```python
from build123d import *

# Parameters (mm, degrees)
PAD_DEPTH    = 22
SKETCH001_R  = 2
POCKET_DEPTH = 15.001


with BuildPart() as part:
    # Sketch → Pad (new body)
    with BuildSketch(Plane.XZ):
        Polygon((0, 0), (28, 0), (28, 35), (18, 35), (18, 15), (0, 15), align=None)
    extrude(amount=PAD_DEPTH)

    # Sketch001 (on Face5 of Pad) → Pocket (cut, through all)
    with BuildSketch(Plane(origin=(0, 0, 15), x_dir=(-1, 0, 0), z_dir=(0, 0, 1))):
        with Locations((-6, 15)):
            Circle(SKETCH001_R)
    extrude(amount=-POCKET_DEPTH, mode=Mode.SUBTRACT)


solid = part.part
```
Verification items for the finished model (mm, model axes). A direction names the side the tool comes from. Give positions to 0.01 mm unless a question says otherwise; leave off trailing zeros. Order: outer loops, then holes, each group sorted by start corner. A loop starts at its lowest first (then second) coordinate and runs counter-clockwise, first axis right, second up. Notation, with made-up numbers: M 29.25,-4.5 L 41.25,-4.5 A23 ccw 41.25,15.5 Z; hole C 27,-24.75 d7. An arc over 180 degrees is marked long. Answer in a Markdown table with one row per item. Add a question column.
Item 1: Mould release check, pull along X, two halves, no side actions. Record for faces 1 (the flat face through (17, 0, 14)), 2 (the flat face through (18, -11, 25)), 3 (the cylindrical face through (6, -17, 8)): released by +X, released by -X, zero draft, split by the parting line, or undercut.
Item 2: Gauge pin test, flat ends, axial feed: pin 1 (2 mm diameter, centred on x = 10.5, y = -13, fed in from +Z); pin 2 (1.5 mm diameter, centred on y = -9.5, z = 31.5, fed in from -X). Record the tip position at first contact, or that the pin passes through.
Item 3: Section check D-D, the plane y = -20. Enter the section's corners in (x, z).
Item 4: Section check A-A, the plane y = -15. Enter the section's corners in (x, z), and give its area (3 significant figures).
Item 5: Section check B-B, the plane x = 6. Enter the section's corners in (y, z), and give its area (3 significant figures).
Item 6: Scan lines: probe 1 along X at (y, z) = (-15, 9.25); probe 2 along Y at (x, z) = (6, 3.75); probe 3 along X at (y, z) = (-3, 28). Record each from-to range of solid material in increasing order. Write a range as from..to.
Item 7: Section check C-C, the plane z = 13.5. Enter the section's corners in (x, y).
Item 8: Tool access check on faces 4 (the flat face through (9, -11, 15)), 5 (the flat face through (0, -11, 8)). Record the directions out of +Z, -Z, +X, -X, +Y, -Y that give a thin tool (end or side, any length) a straight path to the whole face; none if there is none.
Filled sheet:
| question | item | result |
|---|---|---|
| 1 | face 1 | zero draft |
| 1 | face 2 | released by -X |
| 1 | face 3 | undercut |
| 2 | pin 1 | stops at z = 15 |
| 2 | pin 2 | stops at x = 18 |
| 3 | outline | M 0,0 L 28,0 L 28,35 L 18,35 L 18,15 L 0,15 Z |
| 4 | outline | M 0,0 L 4,0 L 4,15 L 0,15 Z; M 8,0 L 28,0 L 28,35 L 18,35 L 18,15 L 8,15 Z |
| 4 | area | 560 mm^2 |
| 5 | outline | M -22,0 L -17,0 L -17,15 L -22,15 Z; M -13,0 L 0,0 L 0,15 L -13,15 Z |
| 5 | area | 270 mm^2 |
| 6 | probe 1 | x = 0..4, 8..28 |
| 6 | probe 2 | y = -22..-17, -13..0 |
| 6 | probe 3 | x = 18..28 |
| 7 | outline | M 0,-22 L 28,-22 L 28,0 L 0,0 Z; hole C 6,-15 d4 |
| 8 | face 4 | +Z, -X, +Y, -Y |
| 8 | face 5 | +Z, -Z, -X, +Y, -Y |
